Autodesk Inventor part; units mm, degrees
ref_plane "YZ Plane" through (0, 0, 0) normal (1, 0, 0) x (0, 1, 0)
ref_plane "XZ Plane" through (0, 0, 0) normal (0, 1, 0) x (-1, 0, 0)
ref_plane "XY Plane" through (0, 0, 0) normal (0, 0, 1) x (1, 0, 0)
sketch "Szkic1" plane through (0, 0, 0) normal (0, 0, 1) x (1, 0, 0)
  line L0 (-1, 0) -> (-14, 0)
  line L1 (-15, 1) -> (-15, 24)
  line L2 (-14, 25) -> (-1, 25)
  line L3 (0, 24) -> (0, 1)
  arc A0 (-14, 25) -> (-15, 24) centre (-14, 24) ccw
  arc A1 (0, 24) -> (-1, 25) centre (-1, 24) ccw
  arc A2 (-1, 0) -> (0, 1) centre (-1, 1) ccw
  arc A3 (-15, 1) -> (-14, 0) centre (-14, 1) ccw
  circle A4 centre (-3, 3) radius 1.5
  circle A5 centre (-12, 3) radius 1.5
  circle A6 centre (-12, 22) radius 1.5
  circle A7 centre (-3, 22) radius 1.5
  line L4 (-3.5, 15) -> (-3.5, 10)
  circle A8 centre (-7.5, 8.5) radius 2
  arc A9 (-3.5, 15) -> (-3.5, 10) centre (-3.5, 12.5) ccw
  point P0 (0, 0)
  point P1 (-15, 25)
  point P2 (-15, 0)
  point P3 (0, 25)
  point P4 (-11.5, 20.5)
  point P5 (-11.5, 4.5)
  point P6 (-3.5, 20.5)
  dimension "d0" = 15
  dimension "d1" = 25
  dimension "d2" = 1
  dimension "d3" = 3
  dimension "d4" = 3
  dimension "d5" = 3
  dimension "d6" = 3
  dimension "d7" = 8
  dimension "d8" = 16
  dimension "d10" = 19
  dimension "d11" = 4
extrude "Wyciągnięcie proste1" add sketch "Szkic1" along normal blind 3
sketch "Szkic2" plane through (0, 0, 3) normal (0, 0, 1) x (1, 0, 0)
  point P0 (0, 0)
sketch "Szkic3" plane through (0, 0, 3) normal (0, 0, 1) x (1, 0, 0)
  point P0 (0, 0)
sketch "Szkic4" plane through (0, 0, 3) normal (0, 0, 1) x (1, 0, 0)
  point P0 (0, 0)
properties part number "zad 7"
Geometry check sheet. Reference: the model listing, model coordinates, mm. A direction names the side the tool comes from. Coordinates: 2 decimals unless noted, no trailing zeros. Write each loop counter-clockwise with the first axis right and the second up, starting at its lowest first coordinate (ties: lowest second). Pieces come first, ordered by that corner, then holes. Notation, with made-up numbers: (73.5, 33) -> (130.5, 33) arc R29 ccw to (130.5, 63) -> close; hole circle Ø3 at (55, 16.5). An arc over 180 degrees is marked (long way). Use CSV: the item, a comma, the result in double quotes. Start each with the question number.
Item 1: Depth check by flat-ended pin: pin 1 Ø2.5 at (x, y) = (-3, 22) entering from -Z. Enter the tip coordinate at first touch or a pass-through.
Item 2: Cross-section at D-D, the plane x = -7.5. Record the cut outline in (y, z), plus the area to 3 significant figures.
Item 3: Mould release check, pull along Y, two halves, no side actions. Record for faces 1 (the cylindrical face through (-14.699, 0.285, 1.479)), 2 (the flat face through (-8, 13, 0)), 3 (the flat face through (-8, 25, 1)), 4 (the cylindrical face through (-9.498, 8.412, 1.479)): released by +Y, released by -Y, zero draft, split by the parting line, or undercut.
Item 4: Cross-section at B-B, the plane x = -3. Record the cut outline in (y, z).
Item 5: Cross-section at A-A, the plane y = 22. Record the cut outline in (x, z).
Item 6: Thickness scan on line 1 (Y direction, x = -12, z = 1.8); line 2 (Y direction, x = -2, z = 0.65); line 3 (Y direction, x = -7.5, z = 1.65). Record the ranges inside material, lowest first.
Item 7: Set-up check for faces 5 (the flat face through (-7, 0, 1)), 6 (the flat face through (-3.5, 13, 1)): record each of +Z, -Z, +X, -X, +Y, -Y from which the full face is reachable in a straight line by a thin tool's end or side.
Item 8: Cross-section at C-C, the plane y = 11. Record the cut outline in (x, z), plus the area to 3 significant figures.
Answers:
1,pin 1,"through"
2,outline,"(0, 0) -> (6.5, 0) -> (6.5, 3) -> (0, 3) -> close; (10.5, 0) -> (25, 0) -> (25, 3) -> (10.5, 3) -> close"
2,area,"63.0 mm^2"
3,face 1,"released by -Y"
3,face 2,"zero draft"
3,face 3,"released by +Y"
3,face 4,"undercut"
4,outline,"(0, 0) -> (1.5, 0) -> (1.5, 3) -> (0, 3) -> close; (4.5, 0) -> (20.5, 0) -> (20.5, 3) -> (4.5, 3) -> close; (23.5, 0) -> (25, 0) -> (25, 3) -> (23.5, 3) -> close"
5,outline,"(-15, 0) -> (-13.5, 0) -> (-13.5, 3) -> (-15, 3) -> close; (-10.5, 0) -> (-4.5, 0) -> (-4.5, 3) -> (-10.5, 3) -> close; (-1.5, 0) -> (0, 0) -> (0, 3) -> (-1.5, 3) -> close"
6,line 1,"0 to 1.5, 4.5 to 20.5, 23.5 to 25"
6,line 2,"0 to 1.88, 4.12 to 20.88, 23.12 to 25"
6,line 3,"0 to 6.5, 10.5 to 25"
7,face 5,"+Z, -Z, +X, -X, -Y"
7,face 6,"+Z, -Z"
8,outline,"(-15, 0) -> (-5.5, 0) -> (-5.5, 3) -> (-15, 3) -> close; (-3.5, 0) -> (0, 0) -> (0, 3) -> (-3.5, 3) -> close"
8,area,"39.0 mm^2"
